```python
from build123d import *

# Parameters (mm, degrees)
F_1_4_CLEARANCE_HOLE1_D = 6.5278
CIRPATTERN1_COUNT       = 6
CHAMFER2_SIZE           = 3.175
SKETCH6_R               = 14.166458521
SKETCH6_R_2             = 12
CUT_EXTRUDE1_DEPTH      = 10
THREAD1_PITCH           = 2


with BuildPart() as part:
    # Sketch1 → Revolve1 (revolve)
    with BuildSketch(Plane.XY, mode=Mode.PRIVATE) as revolve1_sk:
        Polygon((7.5, -49.525), (7.5, -9.006664199), (12.7, 0), (30.48, 0), (30.48, -9.525), (13.5, -9.525), (13.5, -49.525), align=None)
    revolve(revolve1_sk.sketch.rotate(Axis((0, 0, 0), (0, -1, 0)), 90), axis=Axis((0, 0, 0), (0, -1, 0)))

    # 1/4 Clearance Hole1 (through all)
    with Locations(Plane(origin=(0, 0, 0), x_dir=(1, 0, 0), z_dir=(0, 1, 0))):
        with Locations((25.4, 0)):
            f_1_4_clearance_hole1 = Hole(F_1_4_CLEARANCE_HOLE1_D / 2)

    # CirPattern1: 1/4 Clearance Hole1 ×6 about axis
    cirpattern1_axis = Axis((0, 0, 0), (0, 1, 0))
    for i in range(1, CIRPATTERN1_COUNT):
        add(f_1_4_clearance_hole1.rotate(cirpattern1_axis, i * 360 / CIRPATTERN1_COUNT), mode=Mode.SUBTRACT)

    # Chamfer2
    chamfer2_edges = [part.edges().sort_by_distance(p)[0] for p in [
        (0, -9.525, -13.5),
    ]]
    chamfer(chamfer2_edges, length=CHAMFER2_SIZE)

    # Sketch6 → Cut-Extrude1 (cut)
    with BuildSketch(Plane(origin=(0, -49.525, 0), x_dir=(-1, 0, 0), z_dir=(0, -1, 0))):
        Circle(SKETCH6_R)
        with Locations(Location((0, 0, 0), (0, 0, 90))):
            Circle(SKETCH6_R_2, mode=Mode.SUBTRACT)
    extrude(amount=-CUT_EXTRUDE1_DEPTH, mode=Mode.SUBTRACT)

    # Thread1: the profile of Thread Profile2 profile screwed along a right-hand helix of 5 turns, 10 arcs to a turn; built about Z, then put on its axis
    thread1_z = Axis((0, 0, 0), (0, 0, 1))
    thread1_corners = [(12.0003, 0, -0.000173205), (12.0003, 0, 1.7501732), (10.91746825, 0, 1.124999997), (10.91746825, 0, 0.624999997)]
    with BuildLine(mode=Mode.PRIVATE) as thread1_profile:
        Line(thread1_corners[0], thread1_corners[1])
        Line(thread1_corners[1], thread1_corners[2])
        Line(thread1_corners[2], thread1_corners[3])
        Line(thread1_corners[3], thread1_corners[0])
    thread1_cap = Face(thread1_profile.wire())
    thread1_turn_angles = [0, 18, 36, 54, 72, 90, 108, 126, 144, 162, 180, 198, 216, 234, 252, 270, 288, 306, 324, 342, 360]
    thread1_turn_weights = [1, 0.9510565162951535, 1, 0.9510565162951535, 1, 0.9510565162951535, 1, 0.9510565162951535, 1, 0.9510565162951535, 1, 0.9510565162951535, 1, 0.9510565162951535, 1, 0.9510565162951535, 1, 0.9510565162951535, 1, 0.9510565162951535, 1]
    thread1_turn_rails = [Edge.make_bspline([Vector(p[0], p[1], 0).rotate(thread1_z, thread1_turn_angles[k]) / thread1_turn_weights[k] + Vector(0, 0, p[2] + THREAD1_PITCH * thread1_turn_angles[k] / 360) for k in range(21)], [0, 0, 0, 1, 1, 2, 2, 3, 3, 4, 4, 5, 5, 6, 6, 7, 7, 8, 8, 9, 9, 10, 10, 10], 2, thread1_turn_weights) for p in thread1_corners]
    thread1_turn_sides = [Face.make_surface_from_curves(thread1_turn_rails[p[0]], thread1_turn_rails[p[1]]) for p in [(0, 1), (1, 2), (2, 3), (3, 0)]]
    thread1 = Plane(origin=(0, -49.525, 0), x_dir=(1, 0, 0), z_dir=(0, 1, 0)) * Solid(Shell([*[p.moved(Location((0, 0, THREAD1_PITCH * i))) for i in range(5) for p in thread1_turn_sides], thread1_cap, thread1_cap.rotate(thread1_z, 1800).moved(Location((0, 0, THREAD1_PITCH * 1800 / 360)))]))
    add(thread1, mode=Mode.SUBTRACT)


solid = part.part
```
Model file for the job. Use its own axes, mm. A direction names the side the tool comes from. Give positions to 0.01 mm unless a question says otherwise; leave off trailing zeros. Loops run counter-clockwise (first coordinate to the right, second up) from the corner with the lowest first, then second, coordinate; pieces in that order, holes last. Notation, with made-up numbers: M 75,45 L 120,45 A24 cw 120,57 Z; hole C 75.5,33 d1. An arc over 180 degrees is marked long. Use one line per item in the form item = value.
Item 1: Drill centre lines: L1, parallel to Z at x = -25, y = -5; L2, parallel to Y at x = -11, z = 2 (3 decimals); L3, parallel to Z at x = -4.5, y = -2.5. Where is each one in solid material? Low to high.
Filled in:
L1 = -17.44 to -3.24, 3.24 to 17.44
L2 = -49.525 to -47.995, -47.192 to -45.995, -45.192 to -43.995, -43.192 to -41.995, -41.192 to -39.995, -39.192 to -2.632
L3 = -30.15 to -10.32, 10.32 to 30.15
Item 2: Slice it at D-D on y = -16. List the corners of the cut face in (x, z), and give its area (3 significant figures).
Filled in:
outline = C 0,0 d27; hole C 0,0 d15
area = 396 mm^2
Item 3: Two-plate mould, pull along Z, no slides. Class faces 1 (the cylindrical face through (9.44, -4.83, 22.14)), 2 (the cylindrical face through (-30.22, -4.83, -3.97)), 3 (the flat face through (13, -9.525, 13)): released by +Z, released by -Z, zero draft, split by the parting line, or undercut.
Filled in:
face_1 = undercut
face_2 = split by the parting line
face_3 = zero draft
Item 4: Slice it at A-A on y = -4. List the corners of the cut face in (x, z).
Filled in:
outline = C 0,0 d60.96; hole C -25.4,0 d6.53; hole C -12.7,-22 d6.53; hole C -12.7,22 d6.53; hole C 0,0 d20.78; hole C 12.7,-22 d6.53; hole C 12.7,22 d6.53; hole C 25.4,0 d6.53
Item 5: Slice it at C-C on x = 25.4. List the corners of the cut face in (y, z) (3 decimals).
Filled in:
outline = M -9.525,-16.848 L 0,-16.848 L 0,-3.264 L -9.525,-3.264 Z; M -9.525,3.264 L 0,3.264 L 0,16.848 L -9.525,16.848 Z
Item 6: Flat gauge pins, fed straight in: pin 1 Ø4 at (y, z) = (-42, 7) entering from -X; pin 2 Ø6 at (x, z) = (25.4, 0) entering from -Y; pin 3 Ø12 at (x, y) = (-13, -35.5) entering from -Z; pin 4 Ø6 at (x, z) = (1.5, -16.5) entering from +Y. Where does each tip first touch, or does it go through?
Filled in:
pin_1 = -10.89
pin_2 = through
pin_3 = -11.54
pin_4 = 0
Item 7: Which spindle directions (+Z, -Z, +X, -X, +Y, -Y) get a long thin tool onto all of the face, cutting with end or side? Do faces 4 (the flat face through (12, -39.525, 2)), 5 (the cylindrical face through (23.9, -4.8, 2.9)). Say none if no direction does.
Filled in:
face_4 = -Y
face_5 = +Y, -Y
Item 8: Slice it at B-B on z = -20. List the corners of the cut face in (x, y) (3 decimals), and give its area (3 significant figures).
Filled in:
outline = M -23.001,-9.525 L -15.282,-9.525 L -15.282,0 L -23.001,0 Z; M -10.118,-9.525 L 10.118,-9.525 L 10.118,0 L -10.118,0 Z; M 15.282,-9.525 L 23.001,-9.525 L 23.001,0 L 15.282,0 Z
area = 340 mm^2
